Model file for the job. Use its own axes, mm. Face numbers are marked on the shaded views. A direction names the side the tool comes from. Round coordinates to 2 decimals unless told otherwise and drop trailing zeros. Write each loop counter-clockwise with the first axis right and the second up, starting at its lowest first coordinate (ties: lowest second). Pieces come first, ordered by that corner, then holes. Notation, with made-up numbers: (9.5, 87.5) - (23.5, 87.5) arc R9 ccw to (23.5, 94.5) - close; hole circle Ø5 at (-33, 42). An arc over 180 degrees is marked (long way). One line per item, written item: value.
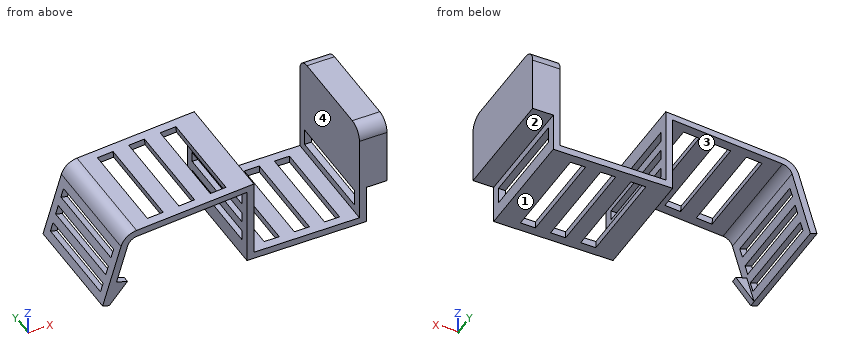
from build123d import *

# Parameters (mm, degrees)
PAD_DEPTH       = 25
SKETCH001_W     = 3.2857142857
SKETCH001_H     = 21
POCKET_DEPTH    = 1.501
SKETCH002_W     = 2.2142857143
SKETCH002_H     = 21
POCKET001_DEPTH = 1.5
SKETCH003_W     = 3.4317132954
SKETCH003_H     = 21
POCKET002_DEPTH = 20.7120716736
SKETCH004_W     = 1.9877118903
SKETCH004_H     = 21
POCKET003_DEPTH = 1.5
FILLET_R        = 3
PAD001_DEPTH    = 1.4
SKETCH006_W     = 3.6
SKETCH006_H     = 21
POCKET004_DEPTH = 6.001


with BuildPart() as part:
    # Sketch → Pad (new body)
    with BuildSketch(Plane.XZ):
        with BuildLine():
            Line((0, 0), (0, -17))
            Line((0, -17), (26, -17))
            Line((26, -17), (26, -8.5))
            Line((26, -8.5), (30.5, -8.5))
            Line((30.5, -8.5), (30.5, 6.5))
            Line((30.5, 6.5), (24.5, 6.5))
            Line((24.5, 6.5), (24.5, -15.5))
            Line((24.5, -15.5), (1.5, -15.5))
            Line((1.5, -15.5), (1.5, 1.5))
            Line((1.5, 1.5), (-24.044265063, -0.50362671))
            ThreePointArc((-24.044265063, -0.50362671), (-26.165331878, -1.347225864), (-27.4385857662, -3.2417992996))
            Line((-27.4385857662, -3.2417992996), (-31.4367394278, -16.5689781716))
            Line((-31.4367394278, -16.5689781716), (-30, -17))
            Line((-30, -17), (-26.0018463384, -3.6728211279))
            ThreePointArc((-23.9389017142, -2), (-25.2281870129, -2.5184722585), (-26.0018463384, -3.6728211279))
            Line((-23.9389017142, -2), (0, 0))
        make_face()
    extrude(amount=PAD_DEPTH)

    # Sketch001 → Pocket (cut, through all)
    with BuildSketch(Plane(origin=(0, 0, -15.5), x_dir=(-1, 0, 0), z_dir=(0, 0, 1))):
        with Locations((-6.4285714286, 12.5)):
            Rectangle(SKETCH001_W, SKETCH001_H)
        with Locations((-13, 12.5)):
            Rectangle(SKETCH001_W, SKETCH001_H)
        with Locations((-19.5714285714, 12.5)):
            Rectangle(SKETCH001_W, SKETCH001_H)
    extrude(amount=-POCKET_DEPTH, mode=Mode.SUBTRACT)

    # Sketch002 → Pocket001 (cut)
    with BuildSketch(Plane(origin=(1.5, 0, 0), x_dir=(0, 0, 1), z_dir=(1, 0, 0))):
        with Locations((-3.3214285714, 12.5)):
            Rectangle(SKETCH002_W, SKETCH002_H)
        with Locations((-7.75, 12.5)):
            Rectangle(SKETCH002_W, SKETCH002_H)
        with Locations((-12.1785714286, 12.5)):
            Rectangle(SKETCH002_W, SKETCH002_H)
    extrude(amount=-POCKET001_DEPTH, mode=Mode.SUBTRACT)

    # Sketch003 → Pocket002 (cut, through all)
    with BuildSketch(Plane(origin=(-0.1077644959, 0, 1.3738910718), x_dir=(-0.9969379064, 0, -0.0781972553), z_dir=(-0.0781972553, 0, 0.9969379064))):
        with Locations((18.8744231246, 12.5)):
            Rectangle(SKETCH003_W, SKETCH003_H)
        with Locations((12.0109965338, 12.5)):
            Rectangle(SKETCH003_W, SKETCH003_H)
        with Locations((5.1475699431, 12.5)):
            Rectangle(SKETCH003_W, SKETCH003_H)
    extrude(amount=-POCKET002_DEPTH, mode=Mode.SUBTRACT)

    # Sketch004 → Pocket003 (cut)
    with BuildSketch(Plane(origin=(-24.2807761251, 0, 7.2842328375), x_dir=(-0.2873478856, 0, -0.9578262852), z_dir=(-0.9578262852, 0, 0.2873478856))):
        with Locations((21.9219155803, 12.5)):
            Rectangle(SKETCH004_W, SKETCH004_H)
        with Locations((17.9464917996, 12.5)):
            Rectangle(SKETCH004_W, SKETCH004_H)
        with Locations((13.9710680189, 12.5)):
            Rectangle(SKETCH004_W, SKETCH004_H)
    extrude(amount=-POCKET003_DEPTH, mode=Mode.SUBTRACT)

    # Fillet
    fillet_edges = [part.edges().sort_by_distance(p)[0] for p in [
        (27.5, -25, 6.5),
        (27.5, 0, 6.5),
    ]]
    fillet(fillet_edges, radius=FILLET_R)

    # Sketch005 → Pad001 (new body)
    with BuildSketch(Plane.XZ.offset(25)):
        Polygon((-28.4195866294, -11.7319554313), (-26.0250209163, -12.4503251452), (-30, -17), align=None)
    extrude(amount=-PAD001_DEPTH)

    # Sketch006 → Pocket004 (cut, through all)
    with BuildSketch(Plane(origin=(24.5, 0, 0), x_dir=(0, 0, -1), z_dir=(-1, 0, 0))):
        with Locations((12, 12.5)):
            Rectangle(SKETCH006_W, SKETCH006_H)
    extrude(amount=-POCKET004_DEPTH, mode=Mode.SUBTRACT)


solid = part.part
1. Band-saw the part on D-D on x = -1. Write the cut outline in (y, z), plus the area to 3 significant figures.
Report:
outline: (-25, -0.08) - (0, -0.08) - (0, 1.3) - (-25, 1.3) - close
area: 34.7 mm²
2. Band-saw the part on A-A on x = -19.5. Write the cut outline in (y, z), plus the area to 3 significant figures.
Report:
outline: (-25, -1.63) - (-23, -1.63) - (-23, -0.15) - (-25, -0.15) - close; (-2, -1.63) - (0, -1.63) - (0, -0.15) - (-2, -0.15) - close
area: 5.93 mm²
3. Tool access for the marked faces 1, 2, 3 and 4: list every direction of +Z, -Z, +X, -X, +Y, -Y with a clear straight run to the whole face (end or side of a thin tool).
Report:
face 1: -Z, +X, -X, +Y, -Y
face 2: -Z, +X, +Y, -Y
face 3: -Z, +Y, -Y
face 4: +Z, +Y, -Y
4. Wall check: probe 1 along X at (y, z) = (-3.75, -6); probe 2 along X at (y, z) = (-17.75, -9.5); probe 3 along Y at (x, z) = (-6, 0). Give the ranges that are in metal, low to high. Write a range as [from, to].
Report:
probe 1: [0, 1.5], [24.5, 30.5]
probe 2: [0, 1.5], [24.5, 26]
probe 3: [-25, -23], [-2, 0]
5. Band-saw the part on C-C on x = -9. Write the cut outline in (y, z).
Report:
outline: (-25, -0.75) - (0, -0.75) - (0, 0.68) - (-25, 0.68) - close
6. Band-saw the part on B-B on y = -7.25. State how many separate pieces and enclosed holes the cut face has, plus the area to 3 significant figures.
Report:
separate pieces: 14
enclosed holes: 0
area: 172 mm²
7. Drop flat-ended pins along their axis: pin 1 (8 mm diameter, centred on x = -19, y = -3, fed in from +Z); pin 2 (5 mm diameter, centred on x = 18, z = -11.5, fed in from +Y); pin 3 (13.5 mm diameter, centred on y = -10.5, z = -6.5, fed in from -X); pin 4 (1.3 mm diameter, centred on x = 27, y = -9, fed in from -Z). Give the stop position or say it passes through.
Report:
pin 1: z = 0.21
pin 2: through
pin 3: x = -30.29
pin 4: z = -8.5
